Input: dimensioned drawing with shaded views. Units: mm. Origin: part minimum x, y, z. A direction names the side the tool comes from. Coordinates: 2 decimals unless noted, no trailing zeros. Order: outer loops, then holes, each group sorted by start corner. A loop starts at its lowest first (then second) coordinate and runs counter-clockwise, first axis right, second up.
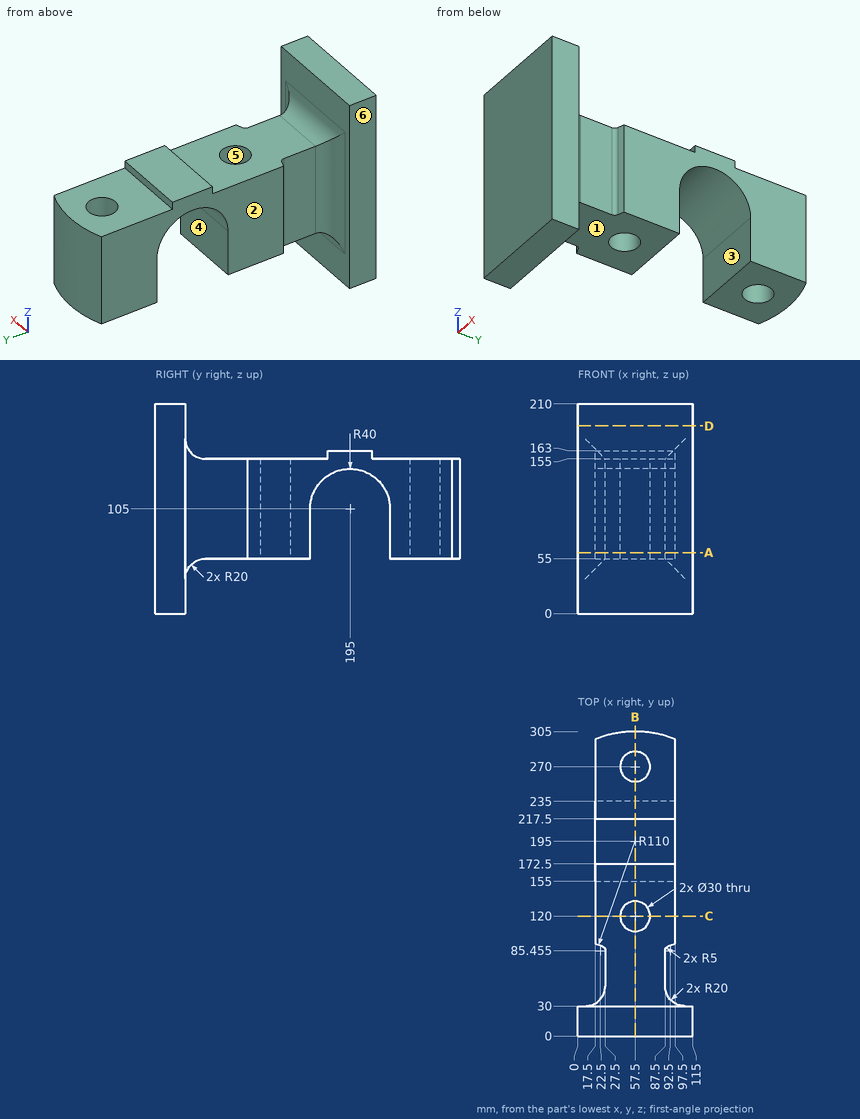
1. Section query D-D on z = 188. Return loops of the section in (x, y), plus the area to 3 significant figures.
Findings:
outline: (0, 0) - (115, 0) - (115, 30) - (0, 30) - close
area: 3,450 mm2
2. Ray query, line 1 (Y direction, x = 57, z = 87); line 2 (X direction, y = 120, z = 120.5); line 3 (Y direction, x = 57.5, z = 123.5) (1 decimal). Return the intervals inside material, ascending.
Findings:
line 1: y = 0 to 105.01, 134.99 to 155, 235 to 255.01, 284.99 to 305
line 2: x = 17.5 to 42.5, 72.5 to 97.5
line 3: y = 0 to 105, 135 to 159.5, 230.5 to 255, 285 to 305
3. Pin query (flat end, axial travel): P1, Ø4, axis at x = 74.5, z = 159.5, coming from the +Y side; P2, Ø13.5, axis at x = 73.5, y = 201, coming from the +Z side; P3, Ø17.5, axis at y = 72, z = 94.5, coming from the -X side; P4, Ø5, axis at x = 93, z = 147.5, coming from the -Y side. Return the tip coordinate at first contact, or that it passes through.
Findings:
P1: stops at y = 217.5
P2: stops at z = 163
P3: stops at x = 27.5
P4: stops at y = 0
4. Section query B-B on x = 57.5. Return loops of the section in (y, z).
Findings:
outline: (0, 0) - (30, 0) - (30, 35) arc R20 cw to (50, 55) - (105, 55) - (105, 155) - (50, 155) arc R20 cw to (30, 175) - (30, 210) - (0, 210) - close; (135, 55) - (155, 55) - (155, 105) arc R40 cw to (235, 105) - (235, 55) - (255, 55) - (255, 155) - (217.5, 155) - (217.5, 163) - (172.5, 163) - (172.5, 155) - (135, 155) - close; (285, 55) - (305, 55) - (305, 155) - (285, 155) - close
5. Access query for the marked faces 1, 2 and 3. Directions: +Z, -Z, +X, -X, +Y, -Y. A direction counts if a zero-diameter tool reaches every point of the face in a straight line with its end or side. Return the directions, or none.
Findings:
face 1: -Z, +X, -X, +Y
face 2: +Z, -Z, -X, +Y
face 3: -Z, +X, -X
6. Draft query along X for the marked faces 4, 5 and 6. Return one class per face: released by +X, released by -X, zero draft, split by the parting line, or undercut.
Findings:
face 4: zero draft
face 5: undercut
face 6: released by -X
7. Section query A-A on z = 61. Return loops of the section in (x, y) (1 decimal), plus the area to 3 significant figures.
Findings:
outline: (0, 0) - (115, 0) - (115, 30) - (107.5, 30) arc R20 cw to (87.5, 50) - (87.5, 85.5) arc R5 cw to (91, 90.2) arc R110 ccw to (97.5, 92.5) - (97.5, 155) - (17.5, 155) - (17.5, 92.5) arc R110 ccw to (24, 90.2) arc R5 cw to (27.5, 85.5) - (27.5, 50) arc R20 cw to (7.5, 30) - (0, 30) - close; (17.5, 235) - (97.5, 235) - (97.5, 297.5) arc R110 ccw to (17.5, 297.5) - close; hole circle Ø30 at (57.5, 120); hole circle Ø30 at (57.5, 270)
area: 16,400 mm2
8. Section query C-C on y = 120. Return loops of the section in (x, z), plus the area to 3 significant figures.
Findings:
outline: (17.5, 55) - (42.5, 55) - (42.5, 155) - (17.5, 155) - close; (72.5, 55) - (97.5, 55) - (97.5, 155) - (72.5, 155) - close
area: 5,000 mm2
